from build123d import *

# Parameters (mm, degrees)
FILLET1_R     = 0.2
CHAMFER1_SIZE = 0.2


with BuildPart() as part:
    # Sketch2 → Revolve1 (revolve)
    with BuildSketch(Plane.XY):
        Polygon((0, 0), (0.875, 0), (0.875, 9), (4, 9), (4, 11), (0, 11), align=None)
    revolve(axis=Axis((0, 11, 0), (0, -1, 0)))

    # Fillet1
    fillet1_edges = [part.edges().sort_by_distance(p)[0] for p in [
        (-0.875, 9, 0),
        (-0.875, 0, 0),
    ]]
    fillet(fillet1_edges, radius=FILLET1_R)

    # Chamfer1
    chamfer1_edges = [part.edges().sort_by_distance(p)[0] for p in [
        (-4, 11, 0),
    ]]
    chamfer(chamfer1_edges, length=CHAMFER1_SIZE)


solid = part.part
Model file for the job. Use its own axes, mm. A direction names the side the tool comes from. Coordinates: 2 decimals unless noted, no trailing zeros. Write each loop counter-clockwise with the first axis right and the second up, starting at its lowest first coordinate (ties: lowest second). Pieces come first, ordered by that corner, then holes. Notation, with made-up numbers: (0.5, 75.25) - (17.5, 75.25) arc R27 ccw to (17.5, 99.25) - close; hole circle Ø11 at (81, 4). An arc over 180 degrees is marked (long way). Write each question's results on one line, items separated by ' | '. Start each with the question number.
1) Cut at A-A (x = 0). Write the cut outline in (y, z) (3 decimals), then the cut area to 3 significant figures.
2) Cut at B-B (z = 0). Write the cut outline in (x, y) (3 decimals), then the cut area to 3 significant figures.
3) 3-axis set-ups, long thin cutter, end or side, ignore diameter. For faces 1 (the face through (0, 0, 0)), 2 (the face through (0.808, 4.56, -0.335)): which of +Z, -Z, +X, -X, +Y, -Y reach the whole face in a straight line?
4) Flat gauge pins, fed straight in: P1, Ø1.5, axis at x = 0, z = 2, coming from the -Y side; P2, Ø3, axis at x = -1.5, y = 7, coming from the +Z side (3 decimals). Where does each tip first touch, or does it go through?
5) Cut at C-C (y = 9.5). Write the cut outline in (x, z), then the cut area to 3 significant figures.
6) Cut at D-D (y = 2.75). Write the cut outline in (x, z) (3 decimals), then the cut area to 3 significant figures.
7) Probe line 1 along Z through (x, y) = (-1.25, 9.5); line 2 along Y through (x, z) = (1.25, -2.75); line 3 along Z through (x, y) = (0, 3) (3 decimals). List the from-to ranges inside material, lowest first. Write a range as from..to.
Returned:
1) outline: (0, -0.675) arc R0.2 ccw to (0.2, -0.875) - (8.8, -0.875) arc R0.2 cw to (9, -1.075) - (9, -4) - (10.8, -4) - (11, -3.8) - (11, 3.8) - (10.8, 4) - (9, 4) - (9, 1.075) arc R0.2 cw to (8.8, 0.875) - (0.2, 0.875) arc R0.2 ccw to (0, 0.675) - close | area: 31.7 mm^2
2) outline: (-4, 9) - (-1.075, 9) arc R0.2 cw to (-0.875, 8.8) - (-0.875, 0.2) arc R0.2 ccw to (-0.675, 0) - (0.675, 0) arc R0.2 ccw to (0.875, 0.2) - (0.875, 8.8) arc R0.2 cw to (1.075, 9) - (4, 9) - (4, 10.8) - (3.8, 11) - (-3.8, 11) - (-4, 10.8) - close | area: 31.7 mm^2
3) face 1: +Z, -Z, +X, -X, -Y | face 2: -Y
4) P1: y = 9 | P2: z = 0.875
5) outline: circle Ø8 at (0, 0) | area: 50.3 mm^2
6) outline: circle Ø1.75 at (0, 0) | area: 2.41 mm^2
7) line 1: -3.8..3.8 | line 2: 9..11 | line 3: -0.875..0.875
